```python
from build123d import *

# Parameters (mm, degrees)
F0_W     = 40
F0_H     = 130
F0_R     = 3.25
F1_DEPTH = 7
F2_W     = 40
F2_H     = 16
F2_R     = 3.25
F3_DEPTH = 5
F4_SIZE  = 2.75
F5_SIZE  = 0.5


with BuildPart() as f1:
    # F0 (on Right) → F1 (new body)
    with BuildSketch(Plane.YZ):
        with Locations((0, 57)):
            Rectangle(F0_W, F0_H)
        with Locations((-13, 0)):
            Circle(F0_R, mode=Mode.SUBTRACT)
        Circle(F0_R, mode=Mode.SUBTRACT)
        with Locations((13, 0)):
            Circle(F0_R, mode=Mode.SUBTRACT)
        with Locations((-13, 114)):
            Circle(F0_R, mode=Mode.SUBTRACT)
        with Locations((0, 114)):
            Circle(F0_R, mode=Mode.SUBTRACT)
        with Locations((13, 114)):
            Circle(F0_R, mode=Mode.SUBTRACT)
    extrude(amount=-F1_DEPTH)

    # F2 (on face) → F3 (join)
    with BuildSketch(Plane.YZ):
        Rectangle(F2_W, F2_H)
        with Locations((-13, 0)):
            Circle(F2_R, mode=Mode.SUBTRACT)
        Circle(F2_R, mode=Mode.SUBTRACT)
        with Locations((13, 0)):
            Circle(F2_R, mode=Mode.SUBTRACT)
    extrude(amount=F3_DEPTH)

    # F4
    f4_edges = [f1.edges().sort_by_distance(p)[0] for p in [
        (-7, -16.25, 0),
        (-7, -3.25, 0),
        (-7, 9.75, 0),
        (-7, 9.75, 114),
        (-7, -3.25, 114),
        (-7, -16.25, 114),
    ]]
    chamfer(f4_edges, length=F4_SIZE)

    # F5
    f5_edges = [f1.edges().sort_by_distance(p)[0] for p in [
        (5, -16.25, 0),
        (5, -3.25, 0),
        (5, 9.75, 0),
        (0, -16.25, 114),
        (0, -3.25, 114),
        (0, 9.75, 114),
    ]]
    chamfer(f5_edges, length=F5_SIZE)


solid = f1.part
```
Can you work these out from the model? Positions are in its coordinate system, mm. Give positions to 0.01 mm unless a question says otherwise; leave off trailing zeros. Write each loop counter-clockwise with the first axis right and the second up, starting at its lowest first coordinate (ties: lowest second). Pieces come first, ordered by that corner, then holes. Notation, with made-up numbers: (-18, 38) -> (6, 38) arc R27 cw to (6, 66) -> close; hole circle Ø6 at (64.25, 28.5). An arc over 180 degrees is marked (long way). Write item = value, one per line.
(1) I need wall thicknesses on probe 1 along Z at (x, y) = (-2.25, -13); probe 2 along Z at (x, y) = (1, 13); probe 3 along Z at (x, y) = (-6.5, 12.5). Which ranges of each line are inside material? Lowest first, please. Write a range as from..to.
Worked out:
probe_1 = -8..-3.25, 3.25..110.75, 117.25..122
probe_2 = -8..-3.25, 3.25..8
probe_3 = -8..-5.48, 5.48..108.52, 119.48..122
(2) Suppose I cut it at B-B on y = 13. Write out the boundary of the cut face in (x, z).
Worked out:
outline = (-7, -8) -> (5, -8) -> (5, -3.75) -> (4.5, -3.25) -> (-4.25, -3.25) -> (-7, -6) -> close; (-7, 6) -> (-4.25, 3.25) -> (4.5, 3.25) -> (5, 3.75) -> (5, 8) -> (0, 8) -> (0, 110.25) -> (-0.5, 110.75) -> (-4.25, 110.75) -> (-7, 108) -> close; (-7, 120) -> (-4.25, 117.25) -> (-0.5, 117.25) -> (0, 117.75) -> (0, 122) -> (-7, 122) -> close
(3) Thinking about a two-plate mould opening in Y: for faces 1 (the face through (-4, 20, 56)), 2 (the face through (-2.349, -0.705, 110.827)), 3 (the face through (-4, -20, 56)), 4 (the face through (-3, 0, 122)), which applies, released by +Y, released by -Y, zero draft, split by the parting line, or undercut?
Worked out:
face_1 = released by +Y
face_2 = undercut
face_3 = released by -Y
face_4 = zero draft
(4) Suppose I cut it at D-D on z = 114. Write out the boundary of the cut face in (x, y), then the cut area to 3 significant figures.
Worked out:
outline = (-7, -20) -> (0, -20) -> (0, -16.75) -> (-0.5, -16.25) -> (-4.25, -16.25) -> (-7, -19) -> close; (-7, -7) -> (-4.25, -9.75) -> (-0.5, -9.75) -> (0, -9.25) -> (0, -3.75) -> (-0.5, -3.25) -> (-4.25, -3.25) -> (-7, -6) -> close; (-7, 6) -> (-4.25, 3.25) -> (-0.5, 3.25) -> (0, 3.75) -> (0, 9.25) -> (-0.5, 9.75) -> (-4.25, 9.75) -> (-7, 7) -> close; (-7, 19) -> (-4.25, 16.25) -> (-0.5, 16.25) -> (0, 16.75) -> (0, 20) -> (-7, 20) -> close
area = 120 mm^2
(5) Suppose I cut it at A-A on z = 0. Write out the boundary of the cut face in (x, y), then the cut area to 3 significant figures.
Worked out:
outline = (-7, -20) -> (5, -20) -> (5, -16.75) -> (4.5, -16.25) -> (-4.25, -16.25) -> (-7, -19) -> close; (-7, -7) -> (-4.25, -9.75) -> (4.5, -9.75) -> (5, -9.25) -> (5, -3.75) -> (4.5, -3.25) -> (-4.25, -3.25) -> (-7, -6) -> close; (-7, 6) -> (-4.25, 3.25) -> (4.5, 3.25) -> (5, 3.75) -> (5, 9.25) -> (4.5, 9.75) -> (-4.25, 9.75) -> (-7, 7) -> close; (-7, 19) -> (-4.25, 16.25) -> (4.5, 16.25) -> (5, 16.75) -> (5, 20) -> (-7, 20) -> close
area = 223 mm^2
(6) I'm going to push flat-ended pins straight in: P1, Ø6, axis at y = -13, z = 0, coming from the +X side; P2, Ø5, axis at y = -0.5, z = 94, coming from the +X side; P3, Ø1.5, axis at x = 3.5, y = 8.5, coming from the +Z side. Where does each tip first touch, or does it pass through?
Worked out:
P1 = through
P2 = 0
P3 = 8
(7) Suppose I cut it at C-C on x = 2.5. Write out the boundary of the cut face in (y, z).
Worked out:
outline = (-20, -8) -> (20, -8) -> (20, 8) -> (-20, 8) -> close; hole circle Ø6.5 at (-13, 0); hole circle Ø6.5 at (0, 0); hole circle Ø6.5 at (13, 0)
